```python
from build123d import *

# Parameters (mm, degrees)
SKETCH1_W                      = 15
SKETCH1_H                      = 15
SKETCH1_R                      = 4.15
BOSS_EXTRUDE1_DEPTH            = 20
SKETCH2_W                      = 15
SKETCH2_H                      = 15
BOSS_EXTRUDE2_DEPTH            = 16
FILLET1_R                      = 5
SKETCH3_R                      = 2.5
CUT_EXTRUDE1_DEPTH             = 4.450447091
CUT_EXTRUDE1_DEPTH_BACK        = 15.930942976
SKETCH4_R                      = 5.25
CUT_EXTRUDE2_DEPTH             = 4.450447091
CUT_EXTRUDE2_DEPTH_BACK        = 7
CUT_EXTRUDE3_REACH             = 39.272
SKETCH5_R                      = 1.6
CUT_EXTRUDE3_DIRECTION_2_DEPTH = 10
CHAMFER1_SIZE                  = 10
CHAMFER1_SIZE2                 = 0.174550649


with BuildPart() as part:
    # Sketch1 → Boss-Extrude1 (new body)
    with BuildSketch(Plane(origin=(0, 0, 0), x_dir=(1, 0, 0), z_dir=(0, 1, 0))):
        Rectangle(SKETCH1_W, SKETCH1_H)
        Circle(SKETCH1_R, mode=Mode.SUBTRACT)
    extrude(amount=BOSS_EXTRUDE1_DEPTH)

    # Sketch2 → Boss-Extrude2 (add)
    with BuildSketch(Plane(origin=(0, 20, 0), x_dir=(1, 0, 0), z_dir=(0, 1, 0))):
        Rectangle(SKETCH2_W, SKETCH2_H)
    extrude(amount=BOSS_EXTRUDE2_DEPTH)

    # Fillet1
    fillet1_edges = [part.edges().sort_by_distance(p)[0] for p in [
        (-7.5, 18, -7.5),
        (7.5, 18, -7.5),
        (7.5, 18, 7.5),
        (-7.5, 18, 7.5),
    ]]
    fillet(fillet1_edges, radius=FILLET1_R)

    # Sketch3 → Cut-Extrude1 (cut, two sides)
    with BuildSketch(Plane(origin=(4.046061336, 0.129475488, 0), x_dir=(0, 0, -1), z_dir=(0.995396198, -0.095845753, 0))) as cut_extrude1_sk:
        with Locations((0, 28.536429083)):
            Circle(SKETCH3_R)
    extrude(amount=CUT_EXTRUDE1_DEPTH, mode=Mode.SUBTRACT)
    extrude(cut_extrude1_sk.sketch, amount=-CUT_EXTRUDE1_DEPTH_BACK, mode=Mode.SUBTRACT)

    # Sketch4 → Cut-Extrude2 (cut, two sides)
    with BuildSketch(Plane(origin=(4.046061336, 0.129475488, 0), x_dir=(0, 0, -1), z_dir=(0.995396198, -0.095845753, 0))) as cut_extrude2_sk:
        with Locations((0, 28.536429083)):
            Circle(SKETCH4_R)
    extrude(amount=CUT_EXTRUDE2_DEPTH, mode=Mode.SUBTRACT)
    extrude(cut_extrude2_sk.sketch, amount=-CUT_EXTRUDE2_DEPTH_BACK, mode=Mode.SUBTRACT)

    # Sketch5 → Cut-Extrude3 (cut, up to next)
    with BuildSketch(Plane(origin=(15.282832762, 35.250598441, 0), x_dir=(-0.995396198, 0.095845753, 0), z_dir=(-0.095845753, -0.995396198, 0)), mode=Mode.PRIVATE) as cut_extrude3_sk1:
        with Locations((12.833853497, 0)):
            Circle(SKETCH5_R)
    cut_extrude3_tool1 = extrude(cut_extrude3_sk1.sketch, amount=CUT_EXTRUDE3_REACH, mode=Mode.PRIVATE) & part.part
    add(cut_extrude3_tool1.solids().sort_by_distance((2.508064, 36.480669, 0))[0], mode=Mode.SUBTRACT)

    # Sketch5 → Cut-Extrude3 direction 2 (cut)
    with BuildSketch(Plane(origin=(15.282832762, 35.250598441, 0), x_dir=(-0.995396198, 0.095845753, 0), z_dir=(-0.095845753, -0.995396198, 0))):
        with Locations((12.833853497, 0)):
            Circle(SKETCH5_R)
    extrude(amount=-CUT_EXTRUDE3_DIRECTION_2_DEPTH, mode=Mode.SUBTRACT)

    # Chamfer1
    chamfer1_edges = [part.edges().sort_by_distance(p)[0] for p in [
        (-4.15, 20, 0),
    ]]
    chamfer1_side = [part.faces().sort_by_distance(p)[0] for p in [
        (-4.15, 10, 0),
    ]]
    chamfer(chamfer1_edges, length=CHAMFER1_SIZE, length2=CHAMFER1_SIZE2, reference=chamfer1_side[0])


solid = part.part
```
Geometry: final body of the model. Coordinates: model frame, mm. A direction names the side the tool comes from. Coordinates: 2 decimals unless noted, no trailing zeros. Order: outer loops, then holes, each group sorted by start corner. A loop starts at its lowest first (then second) coordinate and runs counter-clockwise, first axis right, second up. Notation, with made-up numbers: (76.5, 85.25) - (90.5, 85.25) arc R20 cw to (90.5, 123.25) - close; hole circle Ø7 at (-29, 26). An arc over 180 degrees is marked (long way). Write each question's results on one line, items separated by ' | '.
(1) Set-up query: faces 1 (the face through (-0.9, 4.93, 4.05)), 2 (the face through (3.526, 24.169, -2.423)). Return all of +Z, -Z, +X, -X, +Y, -Y with unobstructed straight access to the full face (end or side cutting, diameter ignored); none if empty.
Values found:
face 1: -Y | face 2: none
(2) Section query D-D, the plane z = 0. Count the separate pieces of the cut face and the enclosed holes in it, plus the area to 3 significant figures.
Values found:
separate pieces: 3 | enclosed holes: 0 | area: 252 mm²
(3) Line query: line 1 (X direction, y = 2.5, z = 0); line 2 (Z direction, x = -1.25, y = 5). Output: solid intervals per line, ascending. Write a range as [from, to].
Values found:
line 1: x = [-7.5, -4.15], [4.15, 7.5] | line 2: z = [-7.5, -3.96], [3.96, 7.5]
(4) First-contact query: pin 1 Ø8 at (x, y) = (4.5, 18.5) entering from +Z; pin 2 Ø2.5 at (x, z) = (-2, 1.5) entering from -Y. Flat tips, straight axial feed; report the tip coordinate or a pass-through.
Values found:
pin 1: stops at z = 7.5 | pin 2: stops at y = 20
(5) Section query A-A, the plane y = 7. Return the cut outline in (x, z).
Values found:
outline: (-7.5, -2.5) arc R5 ccw to (-2.5, -7.5) - (2.5, -7.5) arc R5 ccw to (7.5, -2.5) - (7.5, 2.5) arc R5 ccw to (2.5, 7.5) - (-2.5, 7.5) arc R5 ccw to (-7.5, 2.5) - close; hole circle Ø8.3 at (0, 0)
(6) Section query B-B, the plane z = 6.5. Return the cut outline in (x, y).
Values found:
outline: (-5.5, 0) - (5.5, 0) - (5.5, 36) - (-5.5, 36) - close
(7) Section query C-C, the plane y = 19. Return the cut outline in (x, z).
Values found:
outline: (-7.5, -2.5) arc R5 ccw to (-2.5, -7.5) - (2.5, -7.5) arc R5 ccw to (7.5, -2.5) - (7.5, 2.5) arc R5 ccw to (2.5, 7.5) - (-2.5, 7.5) arc R5 ccw to (-7.5, 2.5) - close; hole circle Ø7.99 at (0, 0)
(8) Mould query, pull axis X, two halves, no side actions, for faces 3 (the face through (-7.5, 34, 0)), 4 (the face through (0, 20, 0)), 5 (the face through (0, 18, -7.5)). Classes: +X half, -X half, draft (parallel to the pull), parting line (faces both ways), or undercut.
Values found:
face 3: -X half | face 4: undercut | face 5: draft
